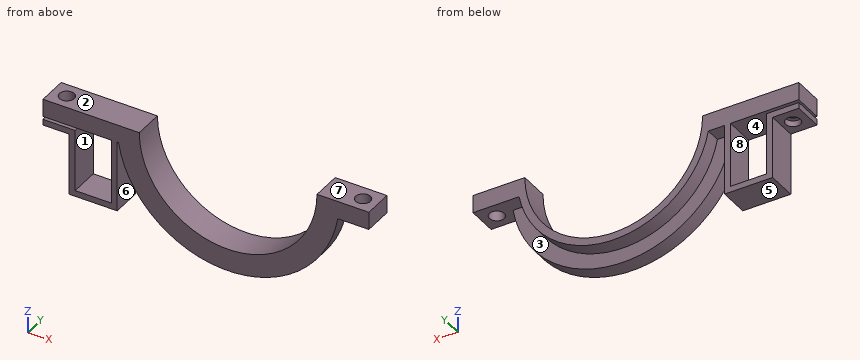
```python
from build123d import *

# Parameters (mm, degrees)
BOSS_EXTRUDE1_DEPTH = 10
BOSS_EXTRUDE2_DEPTH = 5
BOSS_EXTRUDE5_DEPTH = 10
SKETCH3_R           = 2.5
CUT_EXTRUDE4_DEPTH  = 30


with BuildPart() as part:
    # Sketch1 → Boss-Extrude1 (new body)
    with BuildSketch(Plane(origin=(0, 0, 0), x_dir=(1, 0, 0), z_dir=(0, 1, 0))):
        with BuildLine():
            Line((47.5, 6), (31.941352507, 6))
            ThreePointArc((31.941352507, 6), (0, 32.5), (-31.941352507, 6))
            Line((-31.941352507, 6), (-62.5, 6))
            Line((-62.5, 6), (-62.5, 0))
            Line((-62.5, 0), (-30, 0))
            ThreePointArc((-30, 0), (0, 30), (30, 0))
            Line((30, 0), (47.5, 0))
            Line((47.5, 0), (47.5, 6))
        make_face()
    extrude(amount=BOSS_EXTRUDE1_DEPTH)

    # Sketch5 → Boss-Extrude2 (add)
    with BuildSketch(Plane(origin=(0, 0, 0), x_dir=(1, 0, 0), z_dir=(0, 1, 0))):
        with BuildLine():
            ThreePointArc((37.5, 0), (0, 37.5), (-37.5, 0))
            Line((-37.5, 0), (-32.5, 0))
            ThreePointArc((-32.5, 0), (0, 32.5), (32.5, 0))
            Line((32.5, 0), (37.5, 0))
        make_face()
    extrude(amount=BOSS_EXTRUDE2_DEPTH)

    # Sketch1_5 → Boss-Extrude5 (add)
    with BuildSketch(Plane(origin=(0, 0, 0), x_dir=(1, 0, 0), z_dir=(0, 1, 0))):
        Polygon((-39.441352507, 6), (-37.441352507, 6), (-37.441352507, 30), (-53.641352507, 30), (-53.641352507, 9), (-62.5, 9), (-62.5, 7), (-51.641352507, 7), (-51.641352507, 28), (-39.441352507, 28), align=None)
    extrude(amount=BOSS_EXTRUDE5_DEPTH)

    # Sketch3 → Cut-Extrude4 (cut)
    with BuildSketch(Plane.XY):
        with Locations((-57.5, 5)):
            Circle(SKETCH3_R)
        with Locations((42.5, 5)):
            Circle(SKETCH3_R)
    extrude(amount=-CUT_EXTRUDE4_DEPTH, mode=Mode.SUBTRACT)


solid = part.part
```
Design review of the part built by this model. Coordinates are the model's own, in mm. Face numbers are marked on the shaded views. A direction names the side the tool comes from. Give positions to 0.01 mm unless a question says otherwise; leave off trailing zeros. Order: outer loops, then holes, each group sorted by start corner. A loop starts at its lowest first (then second) coordinate and runs counter-clockwise, first axis right, second up. Notation, with made-up numbers: (-18.5, 2) - (30.5, 2) arc R18 cw to (30.5, 26) - close; hole circle Ø7 at (-24, 47.25). An arc over 180 degrees is marked (long way). Use a Markdown table: item, result. Add a question column.
(1) Mouldability with a two-part tool opening along Z and no side actions: class the marked faces 1, 2 and 3 as +Z half, -Z half, draft (parallel to the pull), parting line (faces both ways), or undercut.
(2) Add section B-B on y = 8.5. Give the boundary of the cut face in (x, z).
(3) Add section C-C on x = -57.5. Give the boundary of the cut face in (y, z).
(4) Add section D-D on z = -21.5. Give the boundary of the cut face in (x, y).
(5) Wall thickness on probe 1 along Y at (x, z) = (-57.5, -3.4); probe 2 along Z at (x, y) = (-51, 8.75); probe 3 along X at (y, z) = (3.75, -11.5): over which ranges is each line inside the solid? List them lowest first. Write a range as [from, to].
(6) Clearance check with flat-ended pins moving along their axes: P1, Ø4.5, axis at x = -57.5, y = 5, coming from the +Z side; P2, Ø10, axis at x = -36, z = -20, coming from the -Y side; P3, Ø2.5, axis at x = -56, y = 6.5, coming from the -Z side; P4, Ø2, axis at y = 1.5, z = -30, coming from the +X side (3 decimals). State where each tip first meets the part, or that it passes through.
(7) Machinability: for the marked faces 4, 5, 6, 7 and 8, which of the approach directions +Z, -Z, +X, -X, +Y, -Y give a long, thin tool a straight path to every point of the face, cutting with its end or side? Answer none if there is none.
(8) Add section A-A on x = 42.5. Give the boundary of the cut face in (y, z).
Report:
| question | item | result |
|---|---|---|
| 1 | face 1 | undercut |
| 1 | face 2 | +Z half |
| 1 | face 3 | draft |
| 2 | outline | (-62.5, -9) - (-53.64, -9) - (-53.64, -30) - (-37.44, -30) - (-37.44, -6) - (-31.94, -6) arc R32.5 ccw to (31.94, -6) - (47.5, -6) - (47.5, 0) - (30, 0) arc R30 cw to (-30, 0) - (-62.5, 0) - (-62.5, -6) - (-39.44, -6) - (-39.44, -28) - (-51.64, -28) - (-51.64, -7) - (-62.5, -7) - close |
| 3 | outline | (0, -9) - (2.5, -9) - (2.5, -7) - (0, -7) - close; (0, -6) - (2.5, -6) - (2.5, 0) - (0, 0) - close; (7.5, -9) - (10, -9) - (10, -7) - (7.5, -7) - close; (7.5, -6) - (10, -6) - (10, 0) - (7.5, 0) - close |
| 4 | outline | (-53.64, 0) - (-51.64, 0) - (-51.64, 10) - (-53.64, 10) - close; (-39.44, 0) - (-37.44, 0) - (-37.44, 10) - (-39.44, 10) - close; (-30.72, 0) - (-20.92, 0) - (-20.92, 10) - (-24.37, 10) - (-24.37, 5) - (-30.72, 5) - close; (20.92, 0) - (30.72, 0) - (30.72, 5) - (24.37, 5) - (24.37, 10) - (20.92, 10) - close |
| 5 | probe 1 | y = [0, 2.5], [7.5, 10] |
| 5 | probe 2 | z = [-30, -28], [-6, 0] |
| 5 | probe 3 | x = [-53.64, -51.64], [-39.44, -37.44], [-35.69, -27.71], [27.71, 35.69] |
| 6 | P1 | passes through |
| 6 | P2 | stops at y = 0 |
| 6 | P3 | stops at z = -9 |
| 6 | P4 | stops at x = 23.775 |
| 7 | face 4 | -X, +Y, -Y |
| 7 | face 5 | -Z, -X, +Y, -Y |
| 7 | face 6 | -Z, +Y, -Y |
| 7 | face 7 | +Z, +X, -X, +Y, -Y |
| 7 | face 8 | +Y, -Y |
| 8 | outline | (0, -6) - (2.5, -6) - (2.5, 0) - (0, 0) - close; (7.5, -6) - (10, -6) - (10, 0) - (7.5, 0) - close |
